Design review of the part built by this model. Coordinates are the model's own, in mm. Give positions to 0.01 mm unless a question says otherwise; leave off trailing zeros. Write each loop counter-clockwise with the first axis right and the second up, starting at its lowest first coordinate (ties: lowest second). Pieces come first, ordered by that corner, then holes. Notation, with made-up numbers: (-22.75, 87.25) -> (17.25, 87.25) arc R26 ccw to (17.25, 123.25) -> close; hole circle Ø9 at (-18.5, -6.5). An arc over 180 degrees is marked (long way). Answer as a JSON object with one key per item and string values.
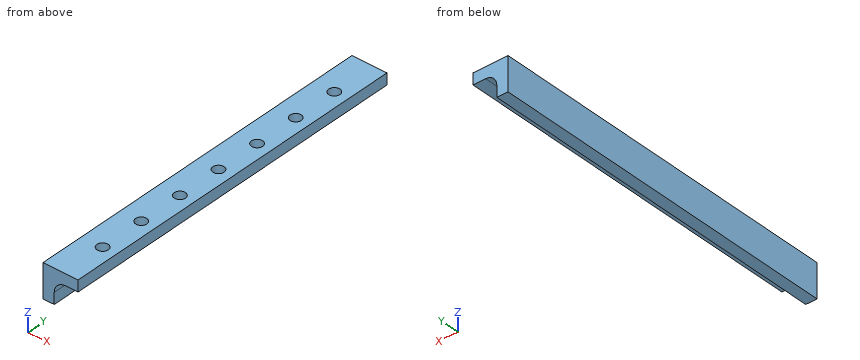
```python
from build123d import *

# Parameters (mm, degrees)
BOSS_EXTRUDE1_DEPTH = 203.2
FILLET1_R           = 6.35
SKETCH2_R           = 3.175
CUT_EXTRUDE1_DEPTH  = 206.050378795
LPATTERN1_COUNT     = 7
LPATTERN1_PITCH     = 25.4


with BuildPart() as part:
    # Sketch1 → Boss-Extrude1 (new body)
    with BuildSketch(Plane(origin=(0, 0, 0), x_dir=(1, 0, 0), z_dir=(0, 1, 0))):
        Polygon((0, 0), (0, 19.05), (6.35, 19.05), (6.35, 6.35), (19.812, 6.35), (19.812, 0), align=None)
    extrude(amount=-BOSS_EXTRUDE1_DEPTH)

    # Fillet1
    fillet1_edges = [part.edges().sort_by_distance(p)[0] for p in [
        (6.35, -101.6, -6.35),
    ]]
    fillet(fillet1_edges, radius=FILLET1_R)

    # Sketch2 → Cut-Extrude1 (cut, through all)
    with BuildSketch(Plane.XY):
        with Locations((11.8745, -25.4)):
            Circle(SKETCH2_R)
    cut_extrude1 = extrude(amount=-CUT_EXTRUDE1_DEPTH, mode=Mode.SUBTRACT)

    # LPattern1: Cut-Extrude1 ×7
    with Locations(*[(0, -i * LPATTERN1_PITCH, 0) for i in range(1, LPATTERN1_COUNT)]):
        add(cut_extrude1, mode=Mode.SUBTRACT)


solid = part.part
```
(1) For line 1 along X through (y, z) = (-25.4, -6); line 2 along X through (y, z) = (-42.5, -17); line 3 along Z through (x, y) = (18.5, -102.5), list the stretches that pass through material, from the lowest coordinate up.
Here are the results:
{"line 1": "x = 0 to 8.7, 15.05 to 19.81", "line 2": "x = 0 to 6.35", "line 3": "z = -6.35 to 0"}
(2) We need section B-B, the plane z = -1.75. Give the number of separate pieces and of enclosed holes in the cut face, then the cut area to 3 significant figures.
Here are the results:
{"separate pieces": "1", "enclosed holes": "7", "area": "3,800 mm²"}
(3) Clearance check with flat-ended pins moving along their axes: pin 1 (5 mm diameter, centred on y = -88, z = -14.5, fed in from +X); pin 2 (7.5 mm diameter, centred on x = 11.87, y = -25.4, fed in from -Z); pin 3 (8.5 mm diameter, centred on x = 11.87, y = -127, fed in from -Z). State where each tip first meets the part, or that it passes through.
Here are the results:
{"pin 1": "stops at x = 6.39", "pin 2": "stops at z = -8.3", "pin 3": "stops at z = -8.89"}
(4) We need section A-A, the plane y = -152.4. State the section outline as (x, z) points.
Here are the results:
{"outline": "(0, -19.05) -> (6.35, -19.05) -> (6.35, -12.7) arc R6.35 cw to (8.7, -7.77) -> (8.7, 0) -> (0, 0) -> close; (15.05, -6.35) -> (19.81, -6.35) -> (19.81, 0) -> (15.05, 0) -> close"}
